Check sheet for the modelled part. Datum: model origin and axes. Units: mm. A direction names the side the tool comes from. Give positions to 0.01 mm unless a question says otherwise; leave off trailing zeros. Order: outer loops, then holes, each group sorted by start corner. A loop starts at its lowest first (then second) coordinate and runs counter-clockwise, first axis right, second up.
```python
from build123d import *

# Parameters (mm, degrees)
BOSS_EXTRUDE1_DEPTH = 5
SKETCH2_R           = 1.95
CUT_EXTRUDE1_DEPTH  = 8
SKETCH3_R           = 1.95
BOSS_EXTRUDE2_DEPTH = 4
FILLET2_START       = -1e-07
FILLET2_OUTLINE_W   = 12
FILLET2_OUTLINE_H   = 5
FILLET2_DEPTH       = 6.0000001
FILLET2_START_2     = -31
FILLET2_2_DEPTH     = 32.804913921
FILLET2_START_3     = 2
FILLET2_3_DEPTH     = 0.9999999
FILLET2_4_OUTLINE_R = 1.95
FILLET2_4_DEPTH     = 3
FILLET3_R           = 0.4


with BuildPart() as part:
    # Sketch1 → Boss-Extrude1 (new body)
    with BuildSketch(Plane(origin=(0, 0, 0), x_dir=(1, 0, 0), z_dir=(0, 1, 0))):
        with BuildLine():
            Line((-6, 0), (-6, 30))
            Line((-6, 30), (6, 30))
            Line((6, 30), (6, 0))
            ThreePointArc((6, 0), (0, -6), (-6, 0))
        make_face()
    extrude(amount=BOSS_EXTRUDE1_DEPTH)

    # Sketch2 → Cut-Extrude1 (cut)
    with BuildSketch(Plane(origin=(0, 0, -30), x_dir=(-1, 0, 0), z_dir=(0, 0, -1))):
        with Locations((0, 2.5)):
            Circle(SKETCH2_R)
    extrude(amount=-CUT_EXTRUDE1_DEPTH, mode=Mode.SUBTRACT)

    # Sketch3 → Boss-Extrude2 (add)
    with BuildSketch(Plane(origin=(0, 5, 0), x_dir=(1, 0, 0), z_dir=(0, 1, 0))):
        with Locations(Location((0, -4.05, 0), (0, 0, 269.999293734))):
            Circle(SKETCH3_R)
    extrude(amount=BOSS_EXTRUDE2_DEPTH)

    # Fillet2: read off the stored shape, not the designer's step
    # Fillet2 outline → Fillet2 (cut)
    with BuildSketch(Plane.XY.offset(FILLET2_START)):
        with Locations((0, 2.5)):
            Rectangle(FILLET2_OUTLINE_W, FILLET2_OUTLINE_H)
    extrude(amount=FILLET2_DEPTH, mode=Mode.SUBTRACT)

    # Fillet2 2 outline → Fillet2 2 (cut)
    with BuildSketch(Plane.XY.offset(FILLET2_START_2)):
        with BuildLine():
            ThreePointArc((-4, 0), (-5.414213562, 0.585786438), (-6, 2))
            Line((-6, 2), (-6, 0))
            Line((-6, 0), (-4, 0))
        make_face()
        with BuildLine():
            Line((-6, 5), (-6, 3))
            ThreePointArc((-6, 3), (-5.414213562, 4.414213562), (-4, 5))
            Line((-4, 5), (-6, 5))
        make_face()
        with BuildLine():
            ThreePointArc((6, 2), (5.414213562, 0.585786438), (4, 0))
            Line((4, 0), (6, 0))
            Line((6, 0), (6, 2))
        make_face()
        with BuildLine():
            Line((6, 5), (4, 5))
            ThreePointArc((4, 5), (5.414213562, 4.414213562), (6, 3))
            Line((6, 3), (6, 5))
        make_face()
    extrude(amount=FILLET2_2_DEPTH, mode=Mode.SUBTRACT)

    # Fillet2 3 outline → Fillet2 3 (add)
    with BuildSketch(Plane(origin=(0, 0, 0), x_dir=(1, 0, 0), z_dir=(0, 1, 0)).offset(FILLET2_START_3)):
        with BuildLine():
            Line((6, 5e-08), (-6, 5e-08))
            ThreePointArc((-6, 5e-08), (0, -6), (6, 5e-08))
        make_face()
    extrude(amount=FILLET2_3_DEPTH)

    # Fillet2 4 outline → Fillet2 4 (add)
    with BuildSketch(Plane(origin=(0, 0, 0), x_dir=(1, 0, 0), z_dir=(0, 1, 0)).offset(FILLET2_START_3)):
        with Locations((0, -4.05)):
            Circle(FILLET2_4_OUTLINE_R)
    extrude(amount=FILLET2_4_DEPTH)

    # Fillet2 5 outline → Fillet2 5 (revolve)
    with BuildSketch(Plane.XY):
        with BuildLine():
            Line((4, 5), (0, 5))
            Line((0, 5), (0, 2.9999999))
            Line((0, 2.9999999), (6, 3))
            ThreePointArc((6, 3), (5.414213562, 4.414213562), (4, 5))
        make_face()
        with BuildLine():
            Line((0, 2), (0, 0))
            Line((0, 0), (4, 0))
            ThreePointArc((4, 0), (5.414213562, 0.585786438), (6, 2))
            Line((6, 2), (0, 2))
        make_face()
    revolve(axis=Axis((0, 0, 0), (0, 1, 0)))

    # Fillet3
    # the kernel refuses this fillet: 0.4 mm, written as the material it takes off along each edge
    with BuildSketch(Plane(origin=(0, 9, 4.05), x_dir=(-1.2326667094924345e-05, 0, 0.9999999999240267), z_dir=(-0.9999999999240267, 0, -1.2326667094924345e-05))) as fillet3_piece_1:
        with BuildLine():
            CenterArc((1.95 - FILLET3_R, -FILLET3_R), FILLET3_R, 0, 90)
            Line((1.95 - FILLET3_R, 0), (1.95, 0))
            Line((1.95, 0), (1.95, -FILLET3_R))
        make_face()
    revolve(axis=Axis((0, 9, 4.05), (0, 1, 0)), mode=Mode.SUBTRACT)


solid = part.part
```
Q1. Tool access check on faces 5 (the flat face through (0, 0, -13)), 6 (the cylindrical face through (0.73, 6.38, 5.86)), 7 (the cylindrical face through (1.547, 1.313, -26.056)). Record the directions out of +Z, -Z, +X, -X, +Y, -Y that give a thin tool (end or side, any length) a straight path to the whole face; none if there is none.
Q2. Sectioned sample at B-B, the plane y = 2.5. Record the cut outline in (x, z), plus the area to 3 significant figures.
Q3. Material ranges on line 1 (Y direction, x = 0, z = -27.5); line 2 (Y direction, x = 2.25, z = -19.5); line 3 (Z direction, x = 4.5, y = 1.5), recorded low to high.
Q4. Sectioned sample at C-C, the plane y = 6.5. Record the cut outline in (x, z).
Q5. Go/stop test with flat-tipped pins: P1, Ø6.5, axis at x = 1.5, z = -11, coming from the +Y side; P2, Ø1.5, axis at x = 0, y = 3.5, coming from the -Z side. Record where each tip stops, or that it passes through.
Q6. Draft check along Y on faces 1 (the flat face through (0, 3, -22)), 2 (the flat face through (6, 2.5, -15.2)), 3 (the cylindrical face through (5.43, 0.6, -15.21)), 4 (the cylindrical face through (-5.43, 4.4, -15.21)). Enter one of: pulls with the +Y half, pulls with the -Y half, needs draft (parallel to the pull), parting line crosses it, or undercut.
Q7. Sectioned sample at A-A, the plane z = -27. Record the cut outline in (x, y).
Filled in:
1. face 5: +Z, -Z, +X, -X, -Y
1. face 6: +Y
1. face 7: -Z
2. outline: (-6, -30) - (-1.95, -30) - (-1.95, -22) - (1.95, -22) - (1.95, -30) - (6, -30) - (6, 0) arc R6 ccw to (-6, 0) - close
2. area: 385 mm2
3. line 1: y = 0 to 0.55, 4.45 to 5
3. line 2: y = 0 to 5
3. line 3: z = -30 to 3.87
4. outline: circle Ø3.9 at (0, 4.05)
5. P1: stops at y = 5
5. P2: stops at z = -22
6. face 1: undercut
6. face 2: needs draft
6. face 3: pulls with the -Y half
6. face 4: pulls with the +Y half
7. outline: (-6, 2) arc R2 ccw to (-4, 0) - (4, 0) arc R2 ccw to (6, 2) - (6, 3) arc R2 ccw to (4, 5) - (-4, 5) arc R2 ccw to (-6, 3) - close; hole circle Ø3.9 at (0, 2.5)
